Part model, mm, in its own coordinate system. Face numbers are marked on the shaded views. A direction names the side the tool comes from. Round coordinates to 2 decimals unless told otherwise and drop trailing zeros. Write each loop counter-clockwise with the first axis right and the second up, starting at its lowest first coordinate (ties: lowest second). Pieces come first, ordered by that corner, then holes. Notation, with made-up numbers: M -27,44 L 25,44 A16 cw 25,74 Z; hole C 47.25,-16 d10. An arc over 180 degrees is marked long. Use one line per item in the form item = value. Start each with the question number.
Item 1: Cut at D-D, the plane y = 119.5. Give the cut face in (x, z), then the cut area to 3 significant figures.
Item 2: Flat gauge pins, fed straight in: pin 1 Ø10 at (y, z) = (65, 39.5) entering from +X; pin 2 Ø10 at (x, z) = (118.5, 20) entering from +Y; pin 3 Ø13.5 at (x, z) = (88, 11.5) entering from -Y. Where does each tip first touch, or does it go through?
Item 3: Cut at A-A, the plane x = 63.5. Give the cut face in (y, z) (3 decimals), then the cut area to 3 significant figures.
Item 4: Cut at B-B, the plane y = 76.2. Give the cut face in (x, z).
Item 5: Probe L1, parallel to Y at x = 63, z = 15; L2, parallel to X at y = 76, z = 14; L3, parallel to Y at x = 117.5, z = 28. List the from-to ranges inside material, lowest first.
Item 6: Mould opens along X. For the marked faces 4, 5, 6 and 7 say: +X half, -X half, draft (parallel to the pull), parting line (faces both ways), or undercut.
Item 7: Which spindle directions (+Z, -Z, +X, -X, +Y, -Y) get a long thin tool onto all of the face, cutting with end or side? Do the marked faces 1, 2 and 3. Say none if no direction does.
Item 8: Cut at C-C, the plane z = 22. Give the cut face in (x, y) (3 decimals), then the cut area to 3 significant figures.
Autodesk Inventor part; units mm, degrees
ref_plane "YZ Plane" through (0, 0, 0) normal (1, 0, 0) x (0, 1, 0)
ref_plane "XZ Plane" through (0, 0, 0) normal (0, 1, 0) x (-1, 0, 0)
ref_plane "XY Plane" through (0, 0, 0) normal (0, 0, 1) x (1, 0, 0)
sketch "Sketch1" plane through (0, 0, 0) normal (0, 0, 1) x (1, 0, 0)
  line L0 (0, 0) -> (12.7, 0)
  line L1 (12.7, 0) -> (12.7, 6.35)
  line L2 (12.7, 6.35) -> (114.3, 6.35)
  line L3 (114.3, 6.35) -> (114.3, 0)
  line L4 (114.3, 0) -> (127, 0)
  line L5 (127, 0) -> (127, 38.1)
  line L6 (127, 38.1) -> (114.3, 38.1)
  line L7 (0, 38.1) -> (12.7, 38.1)
  line L8 (0, 0) -> (0, 76.2)
  line L9 (0, 76.2) -> (63.5, 76.2)
  circle A0 centre (63.5, 76.2) radius 31.75
  arc A1 (114.3, 94.439) -> (12.7, 94.439) centre (63.5, 76.2) ccw
  line L10 (12.7, 38.1) -> (12.7, 94.439)
  line L11 (114.3, 38.1) -> (114.3, 94.439)
  dimension "d0" = 12.7
  dimension "d1" = 6.35
  dimension "d2" = 101.6
  dimension "d3" = 6.35
  dimension "d4" = 12.7
  dimension "d5" = 38.1
  dimension "d6" = 12.7
  dimension "d7" = 38.1
  dimension "d8" = 12.7
  dimension "d9" = 76.2
  dimension "d10" = 63.5
  dimension "d11" = 63.5
  dimension "d12" = 107.95
extrude "Extrusion1" add sketch "Sketch1" along normal blind 44.45 contours L8 L7 L10 A1 L11 L6 L5 L4 L3 L2 L1 L0
properties part number "Assignment 2.5 - Guide Silder"
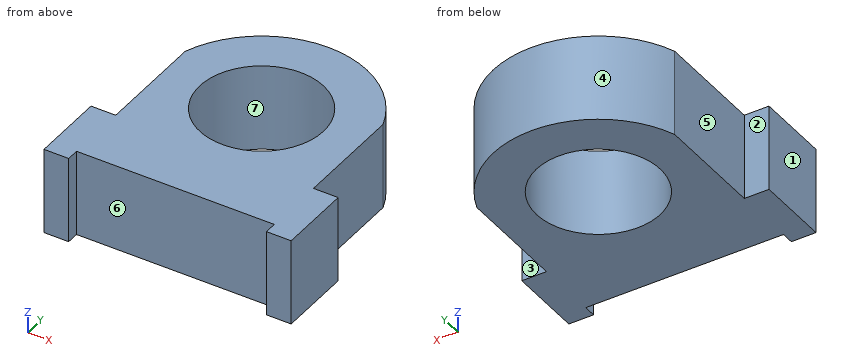
Model answer:
q1.outline = M 31.28,0 L 95.72,0 L 95.72,44.45 L 31.28,44.45 Z
q1.area = 2,860 mm²
q2.pin_1 = 114.3
q2.pin_2 = 96.53
q2.pin_3 = 6.35
q3.outline = M 6.35,0 L 44.45,0 L 44.45,44.45 L 6.35,44.45 Z; M 107.95,0 L 130.175,0 L 130.175,44.45 L 107.95,44.45 Z
q3.area = 2,680 mm²
q4.outline = M 12.7,0 L 31.75,0 L 31.75,44.45 L 12.7,44.45 Z; M 95.25,0 L 114.3,0 L 114.3,44.45 L 95.25,44.45 Z
q5.L1 = 6.35 to 44.45, 107.95 to 130.17
q5.L2 = 12.7 to 31.75, 95.25 to 114.3
q5.L3 = 0 to 38.1
q6.face_4 = parting line
q6.face_5 = -X half
q6.face_6 = undercut
q6.face_7 = undercut
q7.face_1 = +Z, -Z, -X, +Y, -Y
q7.face_2 = +Z, -Z, -X, +Y
q7.face_3 = +Z, -Z, +X, +Y
q8.outline = M 0,0 L 12.7,0 L 12.7,6.35 L 114.3,6.35 L 114.3,0 L 127,0 L 127,38.1 L 114.3,38.1 L 114.3,94.439 A53.975 ccw 12.7,94.439 L 12.7,38.1 L 0,38.1 Z; hole C 63.5,76.2 d63.5
q8.area = 9,400 mm²
